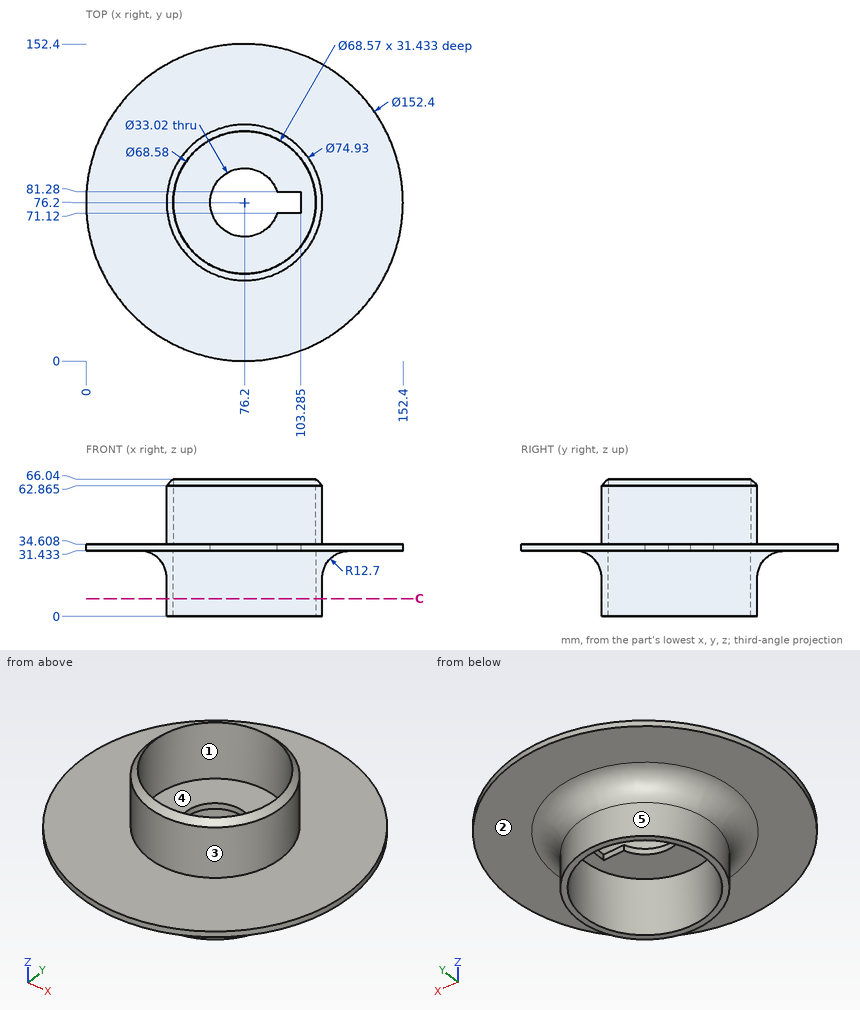
Verification items for this drawing (mm, ordinates from the low corner). A direction names the side the tool comes from. Coordinates: 2 decimals unless noted, no trailing zeros. Write each loop counter-clockwise with the first axis right and the second up, starting at its lowest first coordinate (ties: lowest second). Pieces come first, ordered by that corner, then holes. Notation, with made-up numbers: (43.5, 14) -> (52.5, 14) arc R22 cw to (52.5, 25) -> close; hole circle Ø5 at (49.5, 70.25). An arc over 180 degrees is marked (long way). One line per item, written item: value. Start each with the question number.
Q1. Mould release check, pull along Y, two halves, no side actions. Record for the marked faces 1, 2 and 3: pulls with the +Y half, pulls with the -Y half, needs draft (parallel to the pull), parting line crosses it, or undercut.
Q2. Go/stop test with flat-tipped pins: P1, Ø3.5, axis at x = 99.5, z = 33, coming from the -Y side; P2, Ø1.5, axis at x = 63.5, y = 81.5, coming from the +Z side; P3, Ø1.5, axis at y = 44, z = 36, coming from the -X side; P4, Ø5, axis at x = 20, z = 30, coming from the -Y side. Record where each tip stops, or that it passes through.
Q3. Thickness scan on L1, parallel to Y at x = 76, z = 33; L2, parallel to Y at x = 76, z = 10 (1 decimal). Record the ranges inside material, lowest first. Write a range as from..to.
Q4. Cross-section at C-C on z = 8.5. Enter the section's corners in (x, y) (1 decimal).
Q5. Access from +Z, -Z, +X, -X, +Y, -Y to the whole of each face (thin tool, end or side, straight path). Record for the marked faces 4 and 5.
Checked values:
1. face 1: undercut
1. face 2: needs draft
1. face 3: parting line crosses it
2. P1: stops at y = 3.11
2. P2: passes through
2. P3: stops at x = 55.84
2. P4: stops at y = 22.59
3. L1: y = 0..59.69, 92.71..152.4
3. L2: y = 38.7..41.9, 110.5..113.7
4. outline: circle Ø74.9 at (76.2, 76.2); hole circle Ø68.6 at (76.2, 76.2)
5. face 4: +Z
5. face 5: -Z
